Can you work these out from the model? Positions are in its coordinate system, mm. A direction names the side the tool comes from. Round coordinates to 2 decimals unless told otherwise and drop trailing zeros. Order: outer loops, then holes, each group sorted by start corner. A loop starts at its lowest first (then second) coordinate and runs counter-clockwise, first axis right, second up. Notation, with made-up numbers: (21, -0.75) -> (66, -0.75) arc R27 cw to (66, 22.25) -> close; hole circle Ø8 at (13.25, -36.5). An arc over 180 degrees is marked (long way). One line per item, written item: value.
```python
from build123d import *

# Parameters (mm, degrees)
SKETCH_1_R          = 5
EXTRUDE_1_DEPTH     = 9
SKETCH_2_R          = 2.2
CUT_EXTRUDE_1_DEPTH = 10
SKETCH_3_R          = 0.5
CUT_EXTRUDE_2_DEPTH = 0.2
CHAMFER_1_SIZE      = 0.6


with BuildPart() as part:
    # ｽｹｯﾁ1 → ﾎﾞｽ - 押し出し1 (new body)
    with BuildSketch(Plane(origin=(0, 0, 0), x_dir=(1, 0, 0), z_dir=(0, 1, 0))):
        Circle(SKETCH_1_R)
    extrude(amount=EXTRUDE_1_DEPTH)

    # ｽｹｯﾁ2 → ｶｯﾄ - 押し出し1 (cut, through all)
    with BuildSketch(Plane(origin=(0, 0, 0), x_dir=(1, 0, 0), z_dir=(0, 1, 0))):
        Circle(SKETCH_2_R)
    extrude(amount=CUT_EXTRUDE_1_DEPTH, mode=Mode.SUBTRACT)

    # ｽｹｯﾁ3 → ｶｯﾄ - 押し出し2 (cut)
    with BuildSketch(Plane(origin=(0, 9, 0), x_dir=(1, 0, 0), z_dir=(0, 1, 0))):
        with Locations((0, 3.6)):
            Circle(SKETCH_3_R)
    extrude(amount=-CUT_EXTRUDE_2_DEPTH, mode=Mode.SUBTRACT)

    # 面取り1
    chamfer_1_edges = [part.edges().sort_by_distance(p)[0] for p in [
        (-5, 9, 0),
        (-2.2, 9, 0),
    ]]
    chamfer(chamfer_1_edges, length=CHAMFER_1_SIZE)


solid = part.part
```
Q1. Please list where these lines run through material, in increasing order: line 1 along X through (y, z) = (6.25, 0); line 2 along Z through (x, y) = (0, 8.85); line 3 along Z through (x, y) = (0, 8.9).
Answers below:
line 1: -5 to -2.2, 2.2 to 5
line 2: -4.55 to -4.1, -3.1 to -2.65, 2.65 to 4.55
line 3: -4.5 to -4.1, -3.1 to -2.7, 2.7 to 4.5
Q2. We'd pull the mould along Z, two halves only. Please class faces 1 (the face through (0, 9, 3)), 2 (the face through (2.1, 4.14, -0.66)), 3 (the face through (-1.08, 4.14, 4.88)): released by +Z, released by -Z, zero draft, split by the parting line, or undercut.
Answers below:
face 1: zero draft
face 2: undercut
face 3: split by the parting line
Q3. I want a section at C-C on y = 1.5. List the corners of the cut face in (x, z) for me, plus the area to 3 significant figures.
Answers below:
outline: circle Ø10 at (0, 0); hole circle Ø4.4 at (0, 0)
area: 63.3 mm^2
Q4. I want a section at B-B on x = 0. List the corners of the cut face in (y, z) for me, plus the area to 3 significant figures.
Answers below:
outline: (0, -5) -> (8.4, -5) -> (9, -4.4) -> (9, -4.1) -> (8.8, -4.1) -> (8.8, -3.1) -> (9, -3.1) -> (9, -2.8) -> (8.4, -2.2) -> (0, -2.2) -> close; (0, 2.2) -> (8.4, 2.2) -> (9, 2.8) -> (9, 4.4) -> (8.4, 5) -> (0, 5) -> close
area: 49.5 mm^2
Q5. Will these pins go through, and if not, where does the flat tip stop? pin 1 Ø3 at (x, y) = (-3.5, 4) entering from -Z; pin 2 Ø4 at (x, z) = (0, 0) entering from +Y.
Answers below:
pin 1: z = -4.58
pin 2: through
Q6. On a 3-axis mill with a long thin cutter (end or side, diameter ignored), from which of +Z, -Z, +X, -X, +Y, -Y can I reach the whole of each face in a straight line? I mean faces 4 (the face through (0, 8.8, -3.6)), 5 (the face through (2.2, 0, 1)). Say none if no direction works.
Answers below:
face 4: +Y
face 5: +Z, -Z, +X, -X, -Y
Q7. I want a section at A-A on z = 0. List the corners of the cut face in (x, y) for me, plus the area to 3 significant figures.
Answers below:
outline: (-5, 0) -> (-2.2, 0) -> (-2.2, 8.4) -> (-2.8, 9) -> (-4.4, 9) -> (-5, 8.4) -> close; (2.2, 0) -> (5, 0) -> (5, 8.4) -> (4.4, 9) -> (2.8, 9) -> (2.2, 8.4) -> close
area: 49.7 mm^2
